from build123d import *

# Parameters (mm, degrees)
F0_R     = 1.5875
F1_DEPTH = 2


with BuildPart() as f1:
    # F0 (on Top) → F1 (new body)
    with BuildSketch(Plane.XY):
        with BuildLine():
            ThreePointArc((7.0567981408, -2.54), (7.3883687664, -1.2891884936), (7.5, 0))
            ThreePointArc((7.5, 0), (7.3883687664, 1.2891884936), (7.0567981408, 2.54))
            Line((7.0567981408, 2.54), (0, 2.54))
            Line((0, 2.54), (0, -2.54))
            Line((0, -2.54), (7.0567981408, -2.54))
        make_face()
        with BuildLine():
            ThreePointArc((7.0567981408, 2.54), (7.3883687664, 1.2891884936), (7.5, 0))
            ThreePointArc((7.5, 0), (7.3883687664, -1.2891884936), (7.0567981408, -2.54))
            Line((7.0567981408, -2.54), (38.1, -2.54))
            Line((38.1, -2.54), (38.1, 2.54))
            Line((38.1, 2.54), (7.0567981408, 2.54))
        make_face()
        with BuildLine():
            Line((0, 2.54), (7.0567981408, 2.54))
            ThreePointArc((7.0567981408, 2.54), (-7.5, 0), (7.0567981408, -2.54))
            Line((7.0567981408, -2.54), (0, -2.54))
            Line((0, -2.54), (0, 2.54))
        make_face()
        with Locations((-3.81, 0)):
            Circle(F0_R, mode=Mode.SUBTRACT)
    extrude(amount=F1_DEPTH)


solid = f1.part
Build history of the part. All positions in model axes, mm. A direction names the side the tool comes from. Coordinates: 2 decimals unless noted, no trailing zeros. Order: outer loops, then holes, each group sorted by start corner. A loop starts at its lowest first (then second) coordinate and runs counter-clockwise, first axis right, second up. Notation, with made-up numbers: (-15, 55.25) - (36, 55.25) arc R22 cw to (36, 75.25) - close; hole circle Ø4 at (70.5, 69). An arc over 180 degrees is marked (long way). Write item = value, one per line. Start each with the question number.
1) Saw through at B-B on z = 1.55. Write the cut outline in (x, y) (1 decimal).
2) 3-axis set-ups, long thin cutter, end or side, ignore diameter. For faces 4 (the face through (-7.494, 0.294, 0.986)), 5 (the face through (23, 2.54, 1)): which of +Z, -Z, +X, -X, +Y, -Y reach the whole face in a straight line?
3) Saw through at C-C on x = -3.81. Write the cut outline in (y, z).
4) Saw through at A-A on y = 0. Write the cut outline in (x, z).
5) Two-plate mould, pull along Y, no slides. Class faces 1 (the face through (10, 0, 0)), 2 (the face through (22, -2.54, 1)), 3 (the face through (-5.396, 0.07, 0.986)): pulls with the +Y half, pulls with the -Y half, needs draft (parallel to the pull), parting line crosses it, or undercut.
6) Saw through at D-D on x = 17. Write the cut outline in (y, z).
7) Wall check: line 1 along Y through (x, z) = (30, 0.75); line 2 along X through (y, z) = (1, 0.8); line 3 along Y through (x, z) = (-3.81, 1). Give the ranges that are in metal, low to high. Write a range as from..to.
8) Flat gauge pins, fed straight in: pin 1 Ø0.6 at (x, z) = (27, 1) entering from +Y; pin 2 Ø1 at (x, z) = (30, 1) entering from -Y; pin 3 Ø1 at (y, z) = (1, 1) entering from -X. Where does each tip first touch, or does it go through?
From the geometry:
q1.outline = (7.1, -2.5) - (38.1, -2.5) - (38.1, 2.5) - (7.1, 2.5) arc R7.5 ccw (long way) to start; hole circle Ø3.2 at (-3.8, 0)
q2.face_4 = +Z, -Z
q2.face_5 = +Z, -Z, +X, +Y
q3.outline = (-6.46, 0) - (-1.59, 0) - (-1.59, 2) - (-6.46, 2) - close; (1.59, 0) - (6.46, 0) - (6.46, 2) - (1.59, 2) - close
q4.outline = (-7.5, 0) - (-5.4, 0) - (-5.4, 2) - (-7.5, 2) - close; (-2.22, 0) - (38.1, 0) - (38.1, 2) - (-2.22, 2) - close
q5.face_1 = needs draft
q5.face_2 = pulls with the -Y half
q5.face_3 = undercut
q6.outline = (-2.54, 0) - (2.54, 0) - (2.54, 2) - (-2.54, 2) - close
q7.line_1 = -2.54..2.54
q7.line_2 = -7.43..-5.04, -2.58..38.1
q7.line_3 = -6.46..-1.59, 1.59..6.46
q8.pin_1 = 2.54
q8.pin_2 = -2.54
q8.pin_3 = -7.48
